Geometry: final body of the model. Coordinates: model frame, mm. Face numbers are marked on the shaded views. A direction names the side the tool comes from. Give positions to 0.01 mm unless a question says otherwise; leave off trailing zeros. Loops run counter-clockwise (first coordinate to the right, second up) from the corner with the lowest first, then second, coordinate; pieces in that order, holes last.
1. Section A-A, the plane z = 9. Output: boundary loops of the cut face in (x, y).
2. Material intervals for line 1 along Y through (x, z) = (-73.5, 20); line 2 along Y through (x, z) = (32.5, 11); line 3 along X through (y, z) = (-11, 2.5), sorted ascending.
3. Section B-B, the plane y = 9.5. Output: boundary loops of the cut face in (x, z).
4. First-contact query: P1, Ø1, axis at x = 5.5, z = 8.5, coming from the +Y side; P2, Ø9.5, axis at x = -77, z = 8.5, coming from the +Y side; P3, Ø1, axis at y = -2, z = 28, coming from the +X side. Flat tips, straight axial feed; report the tip coordinate or a pass-through.
5. Access query for the marked faces 1 and 2. Directions: +Z, -Z, +X, -X, +Y, -Y. A direction counts if a zero-diameter tool reaches every point of the face in a straight line with its end or side. Return the directions, or none.
6. Section C-C, the plane x = -68.5. Output: boundary loops of the cut face in (y, z), then the cut area to 3 significant figures.
7. Section D-D, the plane z = 29. Output: boundary loops of the cut face in (x, y).
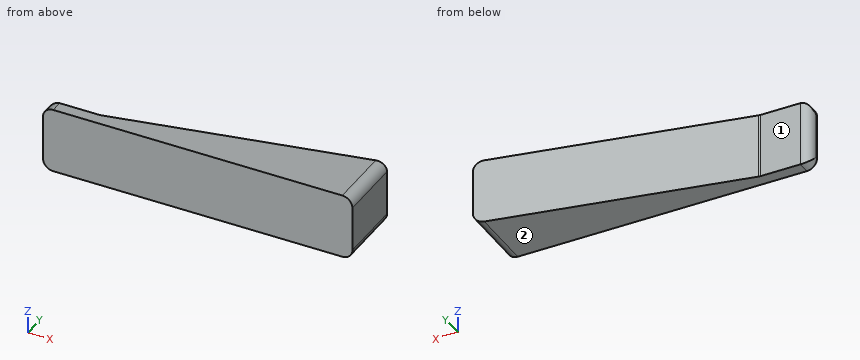
from build123d import *

# Parameters (mm, degrees)
F0_W     = 127
F0_H     = 32
F1_DEPTH = 32
F3_DEPTH = 32
F4_DEPTH = 25
F5_R     = 5


with BuildPart() as f1:
    # F0 (on Top) → F1 (new body)
    with BuildSketch(Plane.XY):
        Rectangle(F0_W, F0_H)
    extrude(amount=F1_DEPTH)

    # F2 (on face) → F3 (cut, through all)
    with BuildSketch(Plane.XY.offset(32)):
        Polygon((-63.5, 16), (-63.5, -10), (63.5, 16), align=None)
    extrude(amount=-F3_DEPTH, mode=Mode.SUBTRACT)

    # F4 (add): a face of the model
    f4_faces = [f1.faces().sort_by_distance(p)[0] for p in [
        (-63.5, -13, 16),
    ]]
    extrude(f4_faces, amount=F4_DEPTH)

    # F5
    f5_edges = [f1.edges().sort_by_distance(p)[0] for p in [
        (63.5, 0, 32),
        (63.5, 0, 0),
        (-63.5, -10, 16),
        (-88.5, -10, 16),
        (-88.5, -13, 32),
        (-88.5, -13, 0),
    ]]
    fillet(f5_edges, radius=F5_R)


solid = f1.part
Answers below:
1. outline: (-88.5, -16) - (63.5, -16) - (63.5, 16) - (-63, -9.9) arc R5 cw to (-64.01, -10) - (-83.5, -10) arc R5 ccw to (-88.5, -15) - close
2. line 1: y = -16 to -10
2. line 2: y = -16 to 9.65
2. line 3: x = -86.5 to 62.83
3. outline: (31.75, 0) - (58.5, 0) arc R5 ccw to (63.5, 5) - (63.5, 27) arc R5 ccw to (58.5, 32) - (31.75, 32) - close
4. P1: stops at y = 4.23
4. P2: stops at y = -10
4. P3: stops at x = 63.47
5. face 1: +Z, -Z, -X, +Y
5. face 2: -Z, +X, -X, +Y, -Y
6. outline: (-16, 0) - (-10, 0) - (-10, 32) - (-16, 32) - close
6. area: 192 mm2
7. outline: (-88.08, -16) - (63.08, -16) - (63.08, 15.91) - (-63, -9.9) arc R5 cw to (-64.01, -10) - (-83.5, -10) arc R5 ccw to (-88.08, -13) - close
